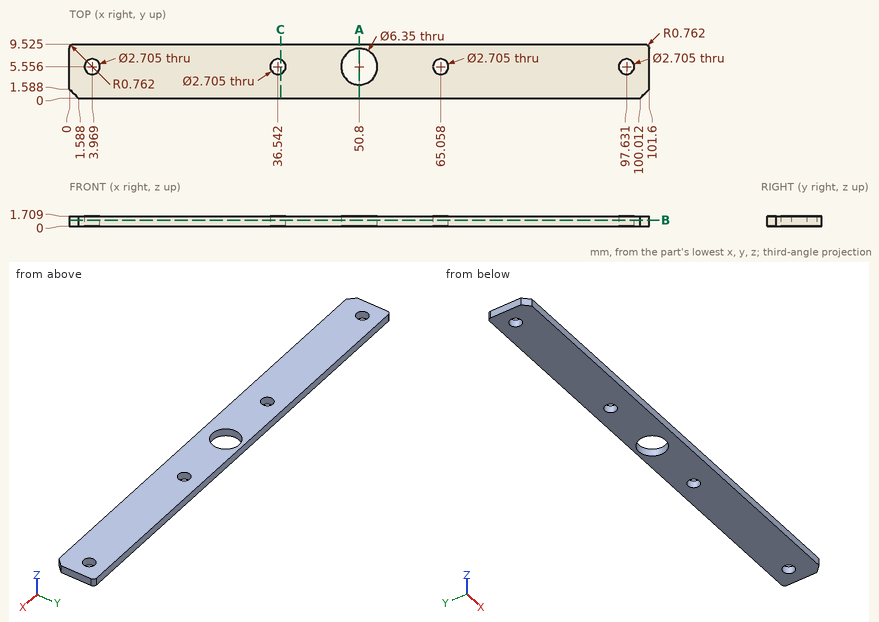
The figure shows three views and two pictorial views of one solid part (mm, origin at its lowest corner). Answer the questions. Round coordinates to 2 decimals unless told otherwise and drop trailing zeros. Loops run counter-clockwise (first coordinate to the right, second up) from the corner with the lowest first, then second, coordinate; pieces in that order, holes last. Notation, with made-up numbers: (56.5, -31.5) - (77.5, -31.5) arc R23 ccw to (77.5, -7.5) - close; hole circle Ø5 at (52.25, 34). An arc over 180 degrees is marked (long way). Use one line per item in the form item = value. Start each with the question number.
(1) Find section C-C on x = 37. Determine the outline of the cut face in (y, z) (1 decimal).
(2) Find section B-B on z = 1.05. Give the number of separate pieces and of enclosed holes in the cut face.
(3) A flat-ended cylindrical pin translates along its axis: P1, Ø2, axis at x = 36.54, y = 5.56, coming from the +Z side. Find the tip coordinate at first contact, or state that the pin passes through.
(4) Consider line 1 (X direction, y = 3.25, z = 1.3) (1 decimal); line 2 (X direction, y = 4, z = 1.15); line 3 (Y direction, x = 37.5, z = 0.3) (1 decimal). Determine where each line is inside the solid, lowest interval first.
(5) Find section A-A on x = 50.8. Determine the outline of the cut face in (y, z) (1 decimal).
Answer list:
q1.outline = (0, 0) - (4.3, 0) - (4.3, 1.7) - (0, 1.7) - close; (6.8, 0) - (9.5, 0) - (9.5, 1.7) - (6.8, 1.7) - close
q2.separate_pieces = 1
q2.enclosed_holes = 5
q3.P1 = through
q4.line_1 = 0 to 48.6, 53 to 101.6
q4.line_2 = 0 to 48.03, 53.57 to 101.6
q4.line_3 = 0 to 4.6, 6.5 to 9.5
q5.outline = (0, 0) - (2.4, 0) - (2.4, 1.7) - (0, 1.7) - close; (8.7, 0) - (9.5, 0) - (9.5, 1.7) - (8.7, 1.7) - close
